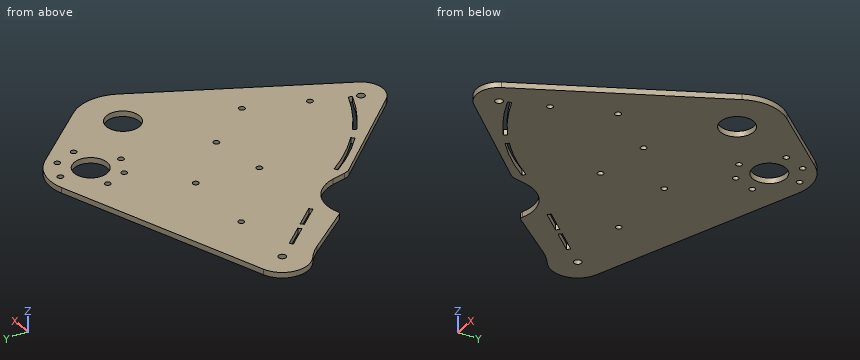
Autodesk Inventor part; units mm, degrees
ref_plane "YZ Plane" through (0, 0, 0) normal (1, 0, 0) x (0, 1, 0)
ref_plane "XZ Plane" through (0, 0, 0) normal (0, 1, 0) x (-1, 0, 0)
ref_plane "XY Plane" through (0, 0, 0) normal (0, 0, 1) x (1, 0, 0)
sketch "Sketch1" plane through (0, 0, 0) normal (0, 0, 1) x (1, 0, 0)
  arc A0 (-7.9109, 20.947) -> (-12.5617, -18.5355) centre (0, 0) ccw
  circle A1 centre (222.25, 0) radius 38.1 construction
  arc A2 (256.45, -16.7919) -> (250.9516, 25.0564) centre (222.25, 0) ccw
  arc A3 (147.4862, -180.0475) -> (178.5388, -175.4733) centre (161.4388, -167.0773) ccw
  line L0 (0, 0) -> (203.2, 0) construction
  line L1 (222.25, 0) -> (161.4388, -167.0773) construction
  line L2 (0, 149.2071) -> (0, -244.4474) construction
  line L3 (-102.8675, 0) -> (329.7763, 0) construction
  line L4 (0, 0) -> (222.25, 0) construction
  circle A4 centre (187.8917, -94.3987) radius 75.057 construction
  circle A5 centre (222.25, 0) radius 25.4 construction
  circle A6 centre (179.1089, 54.2451) radius 25.4 construction
  arc A7 (205.4187, 77.2135) -> (166.7696, 86.9176) centre (179.1089, 54.2451) ccw
  line L5 (205.4187, 77.2135) -> (250.9516, 25.0564)
  line L6 (166.7696, 86.9176) -> (-7.9109, 20.947)
  line L7 (222.25, 0) -> (179.1089, 54.2451) construction
  circle A8 centre (222.25, 0) radius 45.72 construction
  arc A9 (72.7614, -88.5895) -> (32.1142, -67.3414) centre (43.3613, -95.3285) ccw
  line L8 (43.3613, -95.3285) -> (-19.8796, -15.8102) construction
  line L9 (-19.8796, -15.8102) -> (0, 0) construction
  line L10 (28.4453, -66.3716) -> (-1.3022, -28.9676)
  arc A10 (28.4453, -66.3716) -> (32.1142, -67.3414) centre (30.9303, -64.3953) ccw
  arc A11 (-1.3022, -28.9676) -> (-12.5617, -18.5355) centre (-41.0613, -60.588) ccw
  line L11 (72.7614, -88.5895) -> (75.3699, -99.9695)
  line L12 (256.45, -16.7919) -> (178.5388, -175.4733)
  arc A12 (81.8064, -98.3397) -> (163.6106, -161.1103) centre (222.25, 0) ccw
  line L13 (222.25, 0) -> (81.8064, -98.3397) construction
  line L14 (222.25, 0) -> (163.6106, -161.1103) construction
  line L15 (81.8064, -98.3397) -> (84.4072, -96.5186)
  arc A13 (84.4072, -96.5186) -> (164.6966, -158.1268) centre (222.25, 0) ccw
  arc A14 (115.2139, -129.8451) -> (124.5322, -136.9953) centre (222.25, 0) ccw
  line L16 (115.2139, -129.8451) -> (113.1944, -132.295)
  line L17 (124.5322, -136.9953) -> (122.6885, -139.5801)
  line L18 (12.958, -13.9669) -> (46.9467, -51.7215)
  line L19 (25.3128, -32.7489) -> (27.8281, -30.4845)
  line L20 (32.0767, -35.2038) -> (29.5614, -37.4682)
  line L21 (27.8281, -30.4845) -> (32.0767, -35.2038)
  line L22 (10.5984, -16.0912) -> (44.5871, -53.8458)
  line L23 (44.5871, -53.8458) -> (46.9467, -51.7215)
  line L24 (12.958, -13.9669) -> (10.5984, -16.0912)
  line L25 (160.1656, -159.8564) -> (167.0557, -162.3642) construction
  line L26 (167.0557, -162.3642) -> (168.329, -169.5852) construction
  line L27 (168.329, -169.5852) -> (162.7121, -174.2983) construction
  line L28 (162.7121, -174.2983) -> (155.8219, -171.7905) construction
  line L29 (155.8219, -171.7905) -> (154.5487, -164.5695) construction
  line L30 (154.5487, -164.5695) -> (160.1656, -159.8564) construction
  line L31 (161.4388, -167.0773) -> (163.6106, -161.1103) construction
  line L32 (163.6106, -161.1103) -> (164.6966, -158.1268)
  line L33 (147.4862, -180.0475) -> (78.4471, -105.7788)
  arc A15 (75.3699, -99.9695) -> (78.4471, -105.7788) centre (87.7488, -97.132) ccw
  point P0 (193.7916, 35.7832)
  point P1 (-2.1435, -27.9096)
  point P2 (119.8107, -133.5015)
  point P3 (29.9524, -32.8442)
  point P4 (25.4684, -32.6088)
  point P5 (29.717, -37.3281)
  dimension "d30" = 76.2
  dimension "d110" = 91.44
  dimension "d31" = 44.7822
  dimension "d34" = 177.8
  dimension "d39" = 19.05
  dimension "d80" = 22.3911
  dimension "d86" = 222.25
  dimension "d87" = 0
  dimension "d101" = 70
  dimension "d102" = 150.114
  dimension "d103" = 50.8
  dimension "d107" = 69.3086
  dimension "d108" = 59.0923
  dimension "d109" = 34.925
  dimension "d139" = 60.325
  dimension "d140" = 25.4
  dimension "d141" = 101.6
  dimension "d143" = 3.175
  dimension "d176" = 6.35
  dimension "d180" = 171.45
  dimension "d181" = 35
  dimension "d192" = 50.8
  dimension "d194" = 4
  dimension "d195" = 6.35
  dimension "d198" = 50.8
  dimension "d200" = 3.175
  dimension "d201" = 19.05
  dimension "d202" = 3.5
  dimension "d203" = 172.72
  dimension "d204" = 12.7
  dimension "d205" = 168.275
  dimension "d206" = 177.8
  dimension "d216" = 12.7
  dimension "d217" = 150
  dimension "d218" = 101.6
extrude "Extrusion1" add sketch "Sketch1" along normal blind 4.7625 contours L6 A7 L5 A2 L12 A3 L33 A15 L11 A9 A10 L10 A11 A0 | L16 A13 L17 A12 | L18 L20 L22 L19
sketch "Sketch2" plane through (0, 0, 4.7625) normal (0, 0, 1) x (1, 0, 0)
  arc A0 (147.4862, -180.0475) -> (178.5388, -175.4733) centre (161.4388, -167.0773) ccw
  arc A1 (-7.9109, 20.947) -> (-12.5617, -18.5355) centre (0, 0) ccw
  line L0 (178.5388, -175.4733) -> (256.45, -16.7919)
  arc A2 (256.45, -16.7919) -> (250.9516, 25.0564) centre (222.25, 0) ccw
  line L1 (166.7696, 86.9176) -> (-7.9109, 20.947)
  line L2 (250.9516, 25.0564) -> (205.4187, 77.2135)
  arc A3 (205.4187, 77.2135) -> (166.7696, 86.9176) centre (179.1089, 54.2451) ccw
  line L3 (-1.3022, -28.9676) -> (28.4453, -66.3716)
  arc A4 (72.7614, -88.5895) -> (32.1142, -67.3414) centre (43.3613, -95.3285) ccw
  arc A5 (-1.3022, -28.9676) -> (-12.5617, -18.5355) centre (-41.0613, -60.588) ccw
  arc A6 (28.4453, -66.3716) -> (32.1142, -67.3414) centre (30.9303, -64.3953) ccw
  line L4 (72.7614, -88.5895) -> (75.3699, -99.9695)
  arc A7 (75.3699, -99.9695) -> (78.4471, -105.7788) centre (87.7488, -97.132) ccw
  line L5 (78.4471, -105.7788) -> (147.4862, -180.0475)
hole "Structure Holes" at (0, 0, 4.7625) direction (0, 0, -1) diameter 6.35 end through all
sketch "Sketch4" plane through (0, 0, 4.7625) normal (0, 0, 1) x (1, 0, 0)
  arc A0 (147.4862, -180.0475) -> (178.5388, -175.4733) centre (161.4388, -167.0773) ccw
  arc A1 (-7.9109, 20.947) -> (-12.5617, -18.5355) centre (0, 0) ccw
  line L0 (178.5388, -175.4733) -> (256.45, -16.7919)
  arc A2 (256.45, -16.7919) -> (250.9516, 25.0564) centre (222.25, 0) ccw
  line L1 (0, 0) -> (114.3, -50.8) construction
  line L2 (166.7696, 86.9176) -> (-7.9109, 20.947)
  line L3 (250.9516, 25.0564) -> (205.4187, 77.2135)
  arc A3 (205.4187, 77.2135) -> (166.7696, 86.9176) centre (179.1089, 54.2451) ccw
  line L4 (179.1089, 54.2451) -> (271.2167, -45.4479) construction
  line L5 (-1.3022, -28.9676) -> (28.4453, -66.3716)
  arc A4 (72.7614, -88.5895) -> (32.1142, -67.3414) centre (43.3613, -95.3285) ccw
  arc A5 (-1.3022, -28.9676) -> (-12.5617, -18.5355) centre (-41.0613, -60.588) ccw
  arc A6 (28.4453, -66.3716) -> (32.1142, -67.3414) centre (30.9303, -64.3953) ccw
  line L6 (72.7614, -88.5895) -> (75.3699, -99.9695)
  arc A7 (75.3699, -99.9695) -> (78.4471, -105.7788) centre (87.7488, -97.132) ccw
  line L7 (78.4471, -105.7788) -> (147.4862, -180.0475)
  point P0 (153.7287, 55.2488)
  point P1 (160.4527, 37.0083)
  point P2 (178.1052, 28.8649)
  point P3 (196.3456, 35.5888)
  point P4 (204.489, 53.2413)
  point P5 (197.7651, 71.4818)
  point P6 (180.1126, 79.6252)
  point P7 (161.8721, 72.9013)
  dimension "d83" = 114.3
  dimension "d84" = 50.8
  dimension "d132" = 25.4
  dimension "d135" = 360
hole "BearingHole" at (222.25, 0, 4.7625) at (179.1089, 54.2451, 4.7625) direction (0, 0, -1) diameter 28.575 end through all
hole "Hole4" at (114.3, -50.8, 4.7625) direction (0, 0, -1) diameter 5.1054 end through all
sketch "Sketch3" plane through (0, 0, 0) normal (0, 0, -1) x (-1, 0, 0)
  line L0 (0, 0) -> (-222.25, 0) construction
  line L1 (-222.25, 0) -> (-159.267, -173.0444) construction
  line L2 (-84.8185, 0) -> (-175.2456, -129.1434) construction
  line L3 (-130.032, -64.5717) -> (-161.2417, -42.7184) construction
  point P0 (-184.15, 0)
  point P1 (-120.65, 0)
  point P2 (-57.15, 0)
  point P3 (-209.219, -35.8023)
  point P4 (-191.8444, -83.5387)
  point P5 (-174.4698, -131.2751)
  dimension "d10" = 137.4315
  dimension "d11" = 137.4315
  dimension "d12" = 38.1
  dimension "d43" = 38.1
  dimension "d46" = 63.5
  dimension "d51" = 38.1
  dimension "d54" = 50.8
ref_plane "Inner Pitch Plane" through (0, 0, 0) normal (1, 0, 0) x (0, 1, 0)
hole "Hole6" at (180.1126, 79.6252, 4.7625) at (197.7651, 71.4818, 4.7625) at (204.489, 53.2413, 4.7625) at (178.1052, 28.8649, 4.7625) at (160.4527, 37.0083, 4.7625) at (153.7287, 55.2488, 4.7625) direction (0, 0, -1) diameter 4.9784 end through all
hole "Hole8" at (161.2417, -42.7184, 0) at (0, 0, 0) at (222.25, 0, 0) at (120.65, 0, 0) at (57.15, 0, 0) at (191.8444, -83.5387, 0) at (174.4698, -131.2751, 0) direction (0, 0, 1) diameter 5.1054 end through all
hole "Hole9" at (161.4388, -167.0773, 0) direction (0, 0, 1) diameter 6.5278 end through all
equation "\"d10\" = d11"
properties part number "4Bar_Input Side" material "Polycarbonate, Clear"
Read the model definition and answer for the solid it produces. Units are mm, in the model's axes. Coordinates: 2 decimals unless noted, no trailing zeros. Loops run counter-clockwise (first coordinate to the right, second up) from the corner with the lowest first, then second, coordinate; pieces in that order, holes last. Notation, with made-up numbers: (-1, 17) -> (40, 17) arc R28 cw to (40, 40) -> close; hole circle Ø2 at (-16.5, 5.5). An arc over 180 degrees is marked (long way). Return JSON: item names as keys, results as strings.
Item 1: Find section B-B (y = 43.5). Determine the outline of the cut face in (x, z), plus the area to 3 significant figures.
Answers:
{"outline": "(51.81, 0) -> (169.69, 0) -> (169.69, 4.76) -> (51.81, 4.76) -> close; (188.53, 0) -> (234.85, 0) -> (234.85, 4.76) -> (188.53, 4.76) -> close", "area": "782 mm2"}
Item 2: Flat-ended cylindrical pins translate along their axes: P1, Ø4.5, axis at x = 197.77, y = 71.48, coming from the -Z side; P2, Ø1.5, axis at x = 175.5, z = 3, coming from the -Y side (3 decimals); P3, Ø1, axis at y = 20, z = 3, coming from the +X side. Find the tip coordinate at first contact, or state that the pin passes through.
Answers:
{"P1": "passes through", "P2": "stops at y = -180.705", "P3": "stops at x = 254.98"}
Item 3: Find section C-C (z = 2). Count the separate pieces of the cut face and the enclosed holes in it, plus the area to 3 significant figures.
Answers:
{"separate pieces": "1", "enclosed holes": "20", "area": "42,000 mm2"}
Item 4: Find the intervals of material crossed by probe 1 along X at (y, z) = (0, 2.65) (1 decimal); probe 2 along Y at (x, z) = (114.3, 3.35); probe 3 along X at (y, z) = (-101, 0.3), in increasing order.
Answers:
{"probe 1": "x = -22.4 to -3.2, 3.2 to 54.6, 59.7 to 118.1, 123.2 to 208, 236.5 to 260.3", "probe 2": "y = -144.35 to -130.95, -129.09 to -53.35, -48.25 to 67.1", "probe 3": "x = 75.65 to 83.71, 87.66 to 215.1"}
Item 5: Find section A-A (x = 96). Determine the outline of the cut face in (y, z), plus the area to 3 significant figures.
Answers:
{"outline": "(-124.66, 0) -> (-116, 0) -> (-116, 4.76) -> (-124.66, 4.76) -> close; (-111.25, 0) -> (60.19, 0) -> (60.19, 4.76) -> (-111.25, 4.76) -> close", "area": "858 mm2"}
